from build123d import *

# Parameters (mm, degrees)
SKETCH1_R           = 2.5
SKETCH1_W           = 4.3
SKETCH1_H           = 2.3
BOSS_EXTRUDE1_DEPTH = 10
SKETCH2_W           = 4
SKETCH2_H           = 59.39567842
CUT_EXTRUDE1_DEPTH  = 3
FILLET3_R           = 5
CHAMFER2_SIZE       = 4


with BuildPart() as part:
    # Sketch1 → Boss-Extrude1 (new body)
    with BuildSketch(Plane(origin=(0, 0, 0), x_dir=(1, 0, 0), z_dir=(0, 1, 0))):
        Polygon((0, -25), (0, 25), (15, 25), (15, -8), (20, -18), (32, -18), (35, -18), (120, -18), (120, -33), (4, -33), align=None)
        with Locations(Location((5, 20, 0), (0, 0, 270))):
            Circle(SKETCH1_R, mode=Mode.SUBTRACT)
        with Locations(Location((5, -20, 0), (0, 0, 270))):
            Circle(SKETCH1_R, mode=Mode.SUBTRACT)
        with Locations((27.51, -20.72)):
            Rectangle(SKETCH1_W, SKETCH1_H, mode=Mode.SUBTRACT)
    extrude(amount=BOSS_EXTRUDE1_DEPTH)

    # Sketch2 → Cut-Extrude1 (cut)
    with BuildSketch(Plane.XZ):
        with Locations((12, 4.69783921)):
            Rectangle(SKETCH2_W, SKETCH2_H)
    extrude(amount=-CUT_EXTRUDE1_DEPTH, mode=Mode.SUBTRACT)

    # Fillet3
    fillet3_edges = [part.edges().sort_by_distance(p)[0] for p in [
        (120, 5, 33),
        (120, 5, 18),
        (0, 5, -25),
        (15, 5, -25),
    ]]
    fillet(fillet3_edges, radius=FILLET3_R)

    # Chamfer2
    # the kernel refuses this chamfer: 4 mm, written as the material it takes off along each edge
    with BuildSketch(Plane(origin=(20.286731952, 0, 33), x_dir=(0, -0.027495876610586365, -0.9996219169112968), z_dir=(-1, 0, 0))) as chamfer2_piece_1:
        Polygon((CHAMFER2_SIZE * 0.999621916911, -CHAMFER2_SIZE * 0.0274958766106), (-CHAMFER2_SIZE * 0.0274958766106, -CHAMFER2_SIZE * 0.999621916911), (0, 0), align=None)
    extrude(amount=26.573463904, mode=Mode.SUBTRACT)
    with BuildSketch(Plane(origin=(115, 0, 33), x_dir=(0, 0.9996219169112968, 0.02749587661058563), z_dir=(-1, 0, 0))) as chamfer2_piece_2:
        Polygon((CHAMFER2_SIZE * 0.999621916911, CHAMFER2_SIZE * 0.0274958766106), (-CHAMFER2_SIZE * 0.0274958766106, CHAMFER2_SIZE * 0.999621916911), (0, 0), align=None)
    extrude(amount=111.286731952, mode=Mode.SUBTRACT)
    with BuildSketch(Plane(origin=(120, 0, 23), x_dir=(0.02749587661058563, 0.9996219169112968, 0), z_dir=(0, 0, 1))) as chamfer2_piece_3:
        Polygon((CHAMFER2_SIZE * 0.999621916911, CHAMFER2_SIZE * 0.0274958766106), (-CHAMFER2_SIZE * 0.0274958766106, CHAMFER2_SIZE * 0.999621916911), (0, 0), align=None)
    extrude(amount=5, mode=Mode.SUBTRACT)
    with BuildSketch(Plane(origin=(115, 0, 18), x_dir=(0, 0.999621916911297, -0.02749587661058045), z_dir=(-1, 0, 0))) as chamfer2_piece_4_section:
        Polygon((CHAMFER2_SIZE * 0.999621916911, -CHAMFER2_SIZE * 0.0274958766106), (-CHAMFER2_SIZE * 0.0274958766106, -CHAMFER2_SIZE * 0.999621916911), (0, 0), align=None)
    chamfer2_piece_4 = extrude(amount=105.286731952, mode=Mode.PRIVATE)
    chamfer2_piece_4 = split(chamfer2_piece_4, bisect_by=Plane(origin=(30.091205291, 1.322053336, 38.182410583), z_dir=(0.8944271909999159, 0, -0.4472135954999581)), keep=Keep.TOP, mode=Mode.PRIVATE)
    add(chamfer2_piece_4, mode=Mode.SUBTRACT)
    with BuildSketch(Plane(origin=(115, 0, 23), x_dir=(0, 0, -1), z_dir=(-1, 0, 0))) as chamfer2_piece_5:
        Polygon((5, -CHAMFER2_SIZE), (5 - CHAMFER2_SIZE, 0), (5, 0), align=None)
    revolve(axis=Axis((115, 0, 23), (0, -1, 0)), revolution_arc=90, mode=Mode.SUBTRACT)
    with BuildSketch(Plane(origin=(115, 0, 28), x_dir=(0, 0, 1), z_dir=(-1, 0, 0))) as chamfer2_piece_6:
        Polygon((5, CHAMFER2_SIZE), (5 - CHAMFER2_SIZE, 0), (5, 0), align=None)
    revolve(axis=Axis((115, 0, 28), (0, 1, 0)), revolution_arc=90, mode=Mode.SUBTRACT)


solid = part.part
Geometry check sheet. Reference: the model listing, model coordinates, mm. A direction names the side the tool comes from. Round coordinates to 2 decimals unless told otherwise and drop trailing zeros. Loops run counter-clockwise (first coordinate to the right, second up) from the corner with the lowest first, then second, coordinate; pieces in that order, holes last. Notation, with made-up numbers: (16.5, 23.25) -> (43.5, 23.25) arc R18 ccw to (43.5, 53.25) -> close; hole circle Ø10 at (-28, 63). An arc over 180 degrees is marked (long way). Answer as a JSON object with one key per item and string values. Group by question number.
Item 1: Release check for a two-part mould opening along Z. For faces 1 (the face through (61, 0, 24)), 2 (the face through (27, 6, 19.57)), 3 (the face through (59, 2, 31)) record: pulls with the +Z half, pulls with the -Z half, needs draft (parallel to the pull), parting line crosses it, or undercut.
Item 2: Cross-section at B-B, the plane z = -9. Record the cut outline in (x, y).
Item 3: Thickness scan on line 1 along X through (y, z) = (7, -20); line 2 along X through (y, z) = (2, -6.5); line 3 along Z through (x, y) = (90, 5.5). Record the ranges inside material, lowest first.
Item 4: Cross-section at A-A, the plane y = 8.25. Record the cut outline in (x, z).
Item 5: Set-up check for faces 4 (the face through (68, 2, 20)), 5 (the face through (15, 5, -6)), 6 (the face through (12, 3, 4)), 7 (the face through (60, 7, 33)), 8 (the face through (27, 5, 21.87)): record each of +Z, -Z, +X, -X, +Y, -Y from which the full face is reachable in a straight line by a thin tool's end or side.
Item 6: Depth check by flat-ended pin: pin 1 Ø2 at (x, y) = (67.5, 1.5) entering from +Z; pin 2 Ø5 at (y, z) = (7, -3) entering from +X; pin 3 Ø2.5 at (y, z) = (4, 21) entering from +X; pin 4 Ø3 at (x, z) = (5, 20) entering from +Y (3 decimals). Enter the tip coordinate at first touch or a pass-through.
Item 7: Cross-section at C-C, the plane z = 14. Record the cut outline in (x, y).
Determined:
{
 "1": {"face 1": "needs draft", "face 2": "undercut", "face 3": "pulls with the +Z half"},
 "2": {"outline": "(0, 0) -> (10, 0) -> (10, 3) -> (14, 3) -> (14, 0) -> (15, 0) -> (15, 10) -> (0, 10) -> close"},
 "3": {"line 1": "x = 0 to 2.5, 7.5 to 15", "line 2": "x = 0 to 10, 14 to 15", "line 3": "z = 18 to 33"},
 "4": {"outline": "(0, -20) arc R5 ccw to (5, -25) -> (10, -25) arc R5 ccw to (15, -20) -> (15, 8) -> (20, 18) -> (115, 18) arc R5 ccw to (120, 23) -> (120, 28) arc R5 ccw to (115, 33) -> (4, 33) -> (0, 25) -> close; hole circle Ø5 at (5, -20); hole circle Ø5 at (5, 20); hole (25.36, 19.57) -> (29.66, 19.57) -> (29.66, 21.87) -> (25.36, 21.87) -> close"},
 "5": {"face 4": "-Z, +X, -Y", "face 5": "-Z, +X, +Y, -Y", "face 6": "+Z, -Z, -Y", "face 7": "+Z, +X, -X, +Y, -Y", "face 8": "+Y, -Y"},
 "6": {"pin 1": "stops at z = 31.5", "pin 2": "stops at x = 15", "pin 3": "stops at x = 119.94", "pin 4": "passes through"},
 "7": {"outline": "(0, 0) -> (10, 0) -> (10, 3) -> (14, 3) -> (14, 0) -> (18, 0) -> (18, 10) -> (0, 10) -> close"}
}
